from build123d import *

# Parameters (mm, degrees)
SKETCH1_R           = 0.889
SKETCH1_R_2         = 1.75
BOSS_EXTRUDE1_DEPTH = 6
SKETCH2_R           = 1.5
CUT_EXTRUDE1_DEPTH  = 2


with BuildPart() as part:
    # Sketch1 → Boss-Extrude1 (new body)
    with BuildSketch(Plane(origin=(0, 0, 0), x_dir=(1, 0, 0), z_dir=(0, 1, 0))):
        with BuildLine():
            Line((-15.875, 2.5), (-15.875, -2.5))
            Line((-15.875, -2.5), (-4.330127019, -2.5))
            ThreePointArc((-4.330127019, -2.5), (0, -5), (4.330127019, -2.5))
            Line((4.330127019, -2.5), (15.875, -2.5))
            Line((15.875, -2.5), (15.875, 2.5))
            Line((15.875, 2.5), (4.330127019, 2.5))
            ThreePointArc((4.330127019, 2.5), (0, 5), (-4.330127019, 2.5))
            Line((-4.330127019, 2.5), (-15.875, 2.5))
        make_face()
        with Locations(Location((-12.7, 0, 0), (0, 0, 270))):
            Circle(SKETCH1_R, mode=Mode.SUBTRACT)
        with Locations(Location((0, 0, 0), (0, 0, 270))):
            Circle(SKETCH1_R_2, mode=Mode.SUBTRACT)
        with Locations(Location((12.7, 0, 0), (0, 0, 90))):
            Circle(SKETCH1_R, mode=Mode.SUBTRACT)
    extrude(amount=BOSS_EXTRUDE1_DEPTH)

    # Sketch2 → Cut-Extrude1 (cut)
    with BuildSketch(Plane(origin=(0, 6, 0), x_dir=(1, 0, 0), z_dir=(0, 1, 0))):
        with Locations(Location((-12.7, 0, 0), (0, 0, 270))):
            Circle(SKETCH2_R)
        with Locations(Location((12.7, 0, 0), (0, 0, 270))):
            Circle(SKETCH2_R)
    extrude(amount=-CUT_EXTRUDE1_DEPTH, mode=Mode.SUBTRACT)


solid = part.part
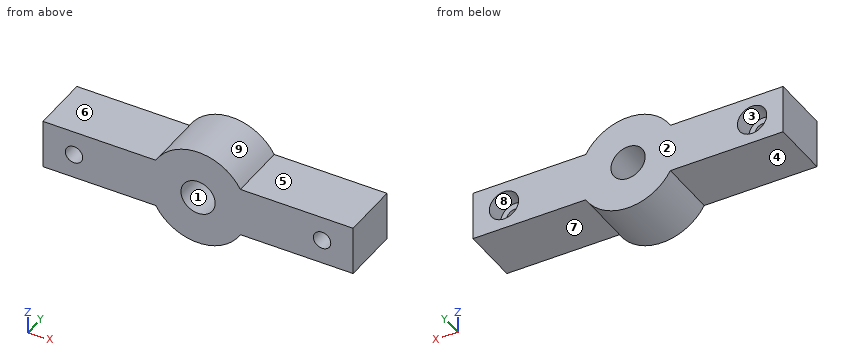
Here's how the part is built. I have some questions about the finished solid (model axes, mm). Face numbers are marked on the shaded views. A direction names the side the tool comes from. Give positions to 0.01 mm unless a question says otherwise; leave off trailing zeros. Order: outer loops, then holes, each group sorted by start corner. A loop starts at its lowest first (then second) coordinate and runs counter-clockwise, first axis right, second up. Notation, with made-up numbers: (18.25, 77) -> (65.25, 77) arc R23 ccw to (65.25, 99) -> close; hole circle Ø10 at (82, -0.75). An arc over 180 degrees is marked (long way). One line per item, written item: value. Start each with the question number.
1. I need wall thicknesses on probe 1 along X at (y, z) = (2.6, 0) (3 decimals); probe 2 along X at (y, z) = (5.55, 0) (3 decimals); probe 3 along Z at (x, y) = (12.7, 1.95). Which ranges of each line are inside material? Lowest first, please. Write a range as from..to.
2. We'd pull the mould along Z, two halves only. Please class the marked faces 1, 2, 3 and 4: released by +Z, released by -Z, zero draft, split by the parting line, or undercut.
3. Imagine slicing it at A-A, the plane x = 12.7. List the corners of the cut face in (y, z) for me, plus the area to 3 significant figures.
4. Imagine slicing it at D-D, the plane x = 0. List the corners of the cut face in (y, z) for me, plus the area to 3 significant figures.
5. Imagine slicing it at B-B, the plane y = 5.2. List the corners of the cut face in (x, z) for me (3 decimals).
6. Imagine slicing it at C-C, the plane z = 0. List the corners of the cut face in (x, y) for me (3 decimals).
7. For the marked faces 5, 6, 7, 8 and 9, which set-ups out of +Z, -Z, +X, -X, +Y, -Y let a thin tool reach every point of the face, with its end or its side?
8. Will these pins go through, and if not, where does the flat tip stop? pin 1 Ø1.5 at (x, z) = (8, 1.5) entering from -Y; pin 2 Ø3 at (x, y) = (-6, 5) entering from +Z; pin 3 Ø1 at (x, y) = (-12.5, 3.5) entering from -Z; pin 4 Ø1.5 at (x, z) = (-13, -0.5) entering from +Y.
Values follow:
1. probe 1: x = -15.875..-13.589, -11.811..-1.75, 1.75..11.811, 13.589..15.875
1. probe 2: x = -15.875..-14.2, -11.2..-1.75, 1.75..11.2, 14.2..15.875
1. probe 3: z = -2.5..-0.89, 0.89..2.5
2. face 1: undercut
2. face 2: zero draft
2. face 3: undercut
2. face 4: released by -Z
3. outline: (0, -2.5) -> (6, -2.5) -> (6, -1.5) -> (4, -1.5) -> (4, -0.89) -> (0, -0.89) -> close; (0, 0.89) -> (4, 0.89) -> (4, 1.5) -> (6, 1.5) -> (6, 2.5) -> (0, 2.5) -> close
3. area: 16.9 mm2
4. outline: (0, -5) -> (6, -5) -> (6, -1.75) -> (0, -1.75) -> close; (0, 1.75) -> (6, 1.75) -> (6, 5) -> (0, 5) -> close
4. area: 39.0 mm2
5. outline: (-15.875, -2.5) -> (-4.33, -2.5) arc R5 ccw to (4.33, -2.5) -> (15.875, -2.5) -> (15.875, 2.5) -> (4.33, 2.5) arc R5 ccw to (-4.33, 2.5) -> (-15.875, 2.5) -> close; hole circle Ø3 at (-12.7, 0); hole circle Ø3.5 at (0, 0); hole circle Ø3 at (12.7, 0)
6. outline: (-15.875, 0) -> (-13.589, 0) -> (-13.589, 4) -> (-14.2, 4) -> (-14.2, 6) -> (-15.875, 6) -> close; (-11.811, 0) -> (-1.75, 0) -> (-1.75, 6) -> (-11.2, 6) -> (-11.2, 4) -> (-11.811, 4) -> close; (1.75, 0) -> (11.811, 0) -> (11.811, 4) -> (11.2, 4) -> (11.2, 6) -> (1.75, 6) -> close; (13.589, 0) -> (15.875, 0) -> (15.875, 6) -> (14.2, 6) -> (14.2, 4) -> (13.589, 4) -> close
7. face 5: +Z, +X, +Y, -Y
7. face 6: +Z, -X, +Y, -Y
7. face 7: -Z, +X, +Y, -Y
7. face 8: +Y
7. face 9: +Z, +Y, -Y
8. pin 1: stops at y = 0
8. pin 2: stops at z = 2.5
8. pin 3: stops at z = -2.5
8. pin 4: stops at y = 4
